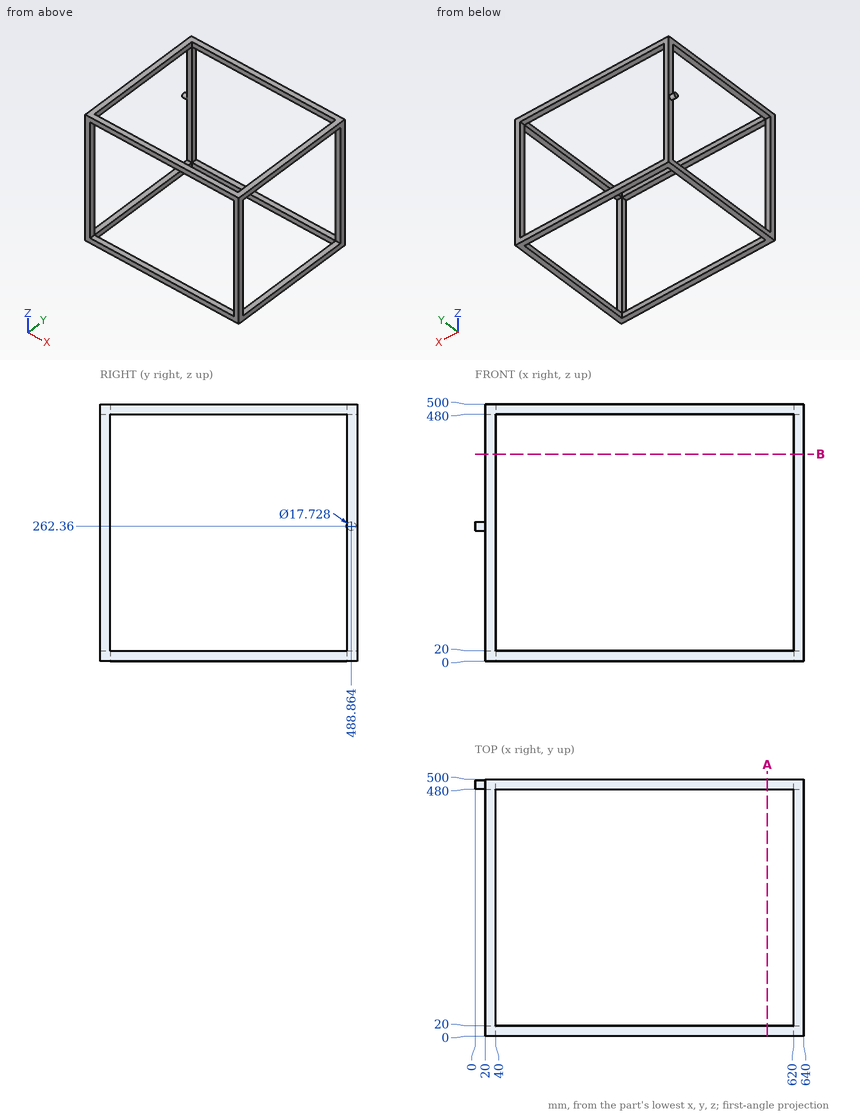
Geometry: see drawing. Coordinates: mm, zero at the bounding-box minimum. Round coordinates to 2 decimals unless told otherwise and drop trailing zeros. Write each loop counter-clockwise with the first axis right and the second up, starting at its lowest first coordinate (ties: lowest second). Pieces come first, ordered by that corner, then holes. Notation, with made-up numbers: (33.5, 2) - (77.5, 2) arc R26 ccw to (77.5, 19) - close; hole circle Ø10 at (1.25, 89.5). An arc over 180 degrees is marked (long way). Use CSV: the item, a comma, the result in double quotes. Start each with the question number.
(1) Cut plane A-A, the plane x = 569. Return loops of the section in (y, z), and give its area (3 significant figures).
(2) First-contact query: pin 1 Ø22 at (y, z) = (489, 331) entering from -X. Flat tip, straight axial feed; report the tip coordinate or a pass-through.
(3) Material intervals for probe 1 along Y at (x, z) = (32, 167.5), sorted ascending. Write a range as [from, to].
(4) Cut plane B-B, the plane z = 402.5. Return loops of the section in (x, y).
Geometry says:
1,outline,"(0, 0) - (20, 0) - (20, 20) - (0, 20) - close; (0, 480) - (20, 480) - (20, 500) - (0, 500) - close; (480, 0) - (500, 0) - (500, 20) - (480, 20) - close; (480, 480) - (500, 480) - (500, 500) - (480, 500) - close"
1,area,"1,600 mm²"
2,pin 1,"x = 20"
3,probe 1,"[0, 20], [480, 500]"
4,outline,"(20, 0) - (40, 0) - (40, 20) - (20, 20) - close; (20, 480) - (40, 480) - (40, 500) - (20, 500) - close; (620, 0) - (640, 0) - (640, 20) - (620, 20) - close; (620, 480) - (640, 480) - (640, 500) - (620, 500) - close"
